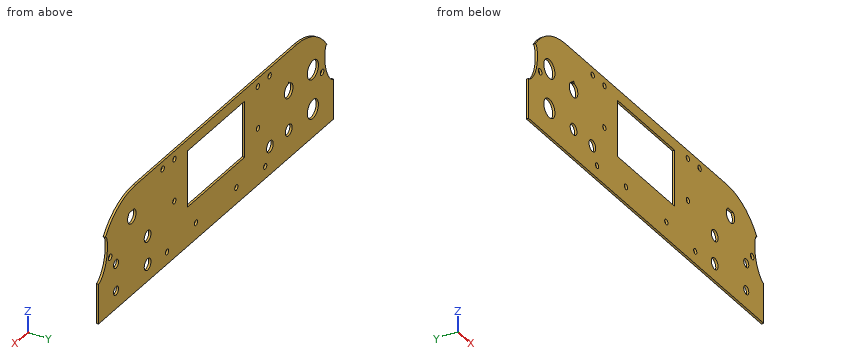
from build123d import *

# Parameters (mm, degrees)
BOSS_EXTRUDE1_DEPTH = 2.54
SKETCH2_W           = 107.95
SKETCH2_H           = 63.5
CUT_EXTRUDE1_DEPTH  = 238.771783963
CUT_EXTRUDE4_START  = -2.54
CUT_EXTRUDE4_DEPTH  = 2.54
SKETCH4_R           = 4.7625
SKETCH4_R_2         = 6.35
SKETCH4_R_3         = 10.5
SKETCH4_R_4         = 3.025
CUT_EXTRUDE3_DEPTH  = 238.771784093
SKETCH6_R           = 3.013751163
SKETCH6_R_2         = 3.176772659
SKETCH6_R_3         = 3.378822927
CUT_EXTRUDE5_DEPTH  = 238.771784093


with BuildPart() as part:
    # Sketch1 → Boss-Extrude1 (new body)
    with BuildSketch(Plane(origin=(0, 0, 0), x_dir=(1, 0, 0), z_dir=(0, 1, 0))):
        with BuildLine():
            Line((222.25, -14.612459999), (222.25, 36.187540001))
            Line((222.25, 36.187540001), (-222.25, 36.187540001))
            Line((-222.25, 36.187540001), (-222.25, -14.612459999))
            ThreePointArc((-222.25, -14.612459999), (-201.791408666, -64.003868664), (-152.4, -84.462459999))
            Line((-152.4, -84.462459999), (152.4, -84.462459999))
            ThreePointArc((152.4, -84.462459999), (201.791408666, -64.003868664), (222.25, -14.612459999))
        make_face()
    extrude(amount=BOSS_EXTRUDE1_DEPTH)

    # Sketch2 → Cut-Extrude1 (cut, through all)
    with BuildSketch(Plane(origin=(0, 2.54, 0), x_dir=(1, 0, 0), z_dir=(0, 1, 0))):
        with Locations((0, -40.012459999)):
            Rectangle(SKETCH2_W, SKETCH2_H)
    extrude(amount=-CUT_EXTRUDE1_DEPTH, mode=Mode.SUBTRACT)

    # Sketch5 → Cut-Extrude4 (cut)
    with BuildSketch(Plane(origin=(0, 2.54, 0), x_dir=(1, 0, 0), z_dir=(0, 1, 0)).offset(CUT_EXTRUDE4_START)):
        with BuildLine():
            ThreePointArc((-222.25, -14.612459999), (-218.970589391, -35.763798683), (-209.440289817, -54.929055063))
            add(Edge.make_bspline(
                [(-209.440289817, -54.929055063), (-204.823931799, -55.506078622), (-202.304901657, -25.266816537), (-219.26819847, -8.373976847), (-222.25, -8.829558466)],
                knots=[0, 0, 0, 0, 0.32580352, 0.516674914, 0.516674914, 0.516674914, 0.516674914], degree=3))
            Line((-222.25, -8.829558466), (-222.25, -14.612459999))
        make_face()
        with BuildLine():
            add(Edge.make_bspline(
                [(-222.25, -8.829558466), (-229.800526338, -9.983183543), (-216.288594077, -54.073048471), (-209.440289817, -54.929055063)],
                knots=[0.516674914, 0.516674914, 0.516674914, 0.516674914, 1, 1, 1, 1], degree=3))
            ThreePointArc((-209.440289817, -54.929055063), (-218.970589391, -35.763798683), (-222.25, -14.612459999))
            Line((-222.25, -14.612459999), (-222.25, -8.829558466))
        make_face()
        with BuildLine():
            add(Edge.make_bspline(
                [(209.440289817, -54.929055063), (204.823931799, -55.506078622), (202.304901657, -25.266816537), (235.136564978, 7.428480335), (216.288594077, -54.073048471), (209.440289817, -54.929055063)],
                knots=[0, 0, 0, 0, 0.32580352, 0.516674914, 1, 1, 1, 1], degree=3))
        make_face()
    extrude(amount=CUT_EXTRUDE4_DEPTH, mode=Mode.SUBTRACT)

    # Sketch4 → Cut-Extrude3 (cut, through all)
    with BuildSketch(Plane(origin=(0, 2.54, 0), x_dir=(1, 0, 0), z_dir=(0, 1, 0))):
        with Locations(Location((189.23, 15.867540001, 0), (0, 0, 270))):
            Circle(SKETCH4_R)
        with Locations(Location((-137.16, 4.437540001, 0), (0, 0, 270))):
            Circle(SKETCH4_R_2)
        with Locations(Location((129.54, 17.137540001, 0), (0, 0, 270))):
            Circle(SKETCH4_R_2)
        with Locations(Location((129.54, -14.612459999, 0), (0, 0, 270))):
            Circle(SKETCH4_R_2)
        with Locations(Location((189.23, -14.612459999, 0), (0, 0, 270))):
            Circle(SKETCH4_R)
        with Locations(Location((-182.88, -40.012459999, 0), (0, 0, 270))):
            Circle(SKETCH4_R_3)
        with Locations(Location((-182.88, 4.437540001, 0), (0, 0, 270))):
            Circle(SKETCH4_R_3)
        with Locations(Location((-101.6, 4.437540001, 0), (0, 0, 270))):
            Circle(SKETCH4_R_2)
        with Locations(Location((-38.130967929, 17.745240001, 0), (0, 0, 270))):
            Circle(SKETCH4_R_4)
        with Locations(Location((-79, -27.947459999, 0), (0, 0, 270))):
            Circle(SKETCH4_R_4)
        with Locations(Location((-78.7827, -75.287459999, 0), (0, 0, 270))):
            Circle(SKETCH4_R_4)
        with Locations(Location((78.7827, -75.287459999, 0), (0, 0, 270))):
            Circle(SKETCH4_R_4)
        with Locations(Location((79, -27.947459999, 0), (0, 0, 270))):
            Circle(SKETCH4_R_4)
        with Locations(Location((38.130967929, 17.745240001, 0), (0, 0, 270))):
            Circle(SKETCH4_R_4)
        with BuildLine():
            Line((-138.01, -48.067737772), (-138.01, -49.812459999))
            Line((-138.01, -49.812459999), (-136.31, -49.812459999))
            Line((-136.31, -49.812459999), (-136.31, -48.067737772))
            ThreePointArc((-136.31, -48.067737772), (-137.16, -31.912459999), (-138.01, -48.067737772))
        make_face()
        with BuildLine():
            Line((164.1475, -59.062459999), (154.6225, -59.062459999))
            ThreePointArc((154.6225, -59.062459999), (159.385, -44.774959999), (164.1475, -59.062459999))
        make_face()
    extrude(amount=-CUT_EXTRUDE3_DEPTH, mode=Mode.SUBTRACT)

    # Sketch6 → Cut-Extrude5 (cut, through all)
    with BuildSketch(Plane.XZ):
        with Locations(Location((92.768348893, -22.335077387, 0), (0, 0, 270))):
            Circle(SKETCH6_R)
        with Locations(Location((101.056164591, 75.862981341, 0), (0, 0, 270))):
            Circle(SKETCH6_R_2)
        with Locations(Location((200.350154748, 27.883658386, 0), (0, 0, 270))):
            Circle(SKETCH6_R_3)
        with Locations(Location((-92.768348893, -22.335077387, 0), (0, 0, 90))):
            Circle(SKETCH6_R)
        with Locations(Location((-200.350154748, 27.883658386, 0), (0, 0, 90))):
            Circle(SKETCH6_R_3)
        with Locations(Location((-101.056164591, 75.862981341, 0), (0, 0, 90))):
            Circle(SKETCH6_R_2)
    extrude(amount=-CUT_EXTRUDE5_DEPTH, mode=Mode.SUBTRACT)


solid = part.part
Source: CAD feature listing. Evaluate the final solid. Frame: model axes, mm. Round coordinates to 2 decimals unless told otherwise and drop trailing zeros. Write each loop counter-clockwise with the first axis right and the second up, starting at its lowest first coordinate (ties: lowest second). Pieces come first, ordered by that corner, then holes. Notation, with made-up numbers: (50.25, 45) - (79.25, 45) arc R20 cw to (79.25, 49) - close; hole circle Ø8 at (1, 74.25). An arc over 180 degrees is marked (long way). Use CSV: the item, a comma, the result in double quotes. Start each with the question number.
(1) Cut plane A-A, the plane x = 189.23. Return loops of the section in (y, z), and give its area (3 significant figures).
(2) Material intervals for probe 1 along Z at (x, y) = (-142, 0.1); probe 2 along X at (y, z) = (2.25, 15) (3 decimals); probe 3 along Z at (x, y) = (-43, 0.95), sorted ascending. Write a range as [from, to].
(3) Cut plane C-C, the plane y = 0.9. Give the number of separate pieces and of enclosed holes in the cut face, and give its area (3 significant figures).
(4) Cut plane B-B, the plane x = -182.88. Return loops of the section in (y, z).
(5) First-contact query: pin 1 Ø0.9 at (y, z) = (2, 49) entering from +X. Flat tip, straight axial feed; report the tip coordinate or a pass-through.
Geometry says:
1,outline,"(0, -36.19) - (2.54, -36.19) - (2.54, -20.63) - (0, -20.63) - close; (0, -11.11) - (2.54, -11.11) - (2.54, 9.85) - (0, 9.85) - close; (0, 19.37) - (2.54, 19.37) - (2.54, 73.96) - (0, 73.96) - close"
1,area,"231 mm²"
2,probe 1,"[-36.19, -8.55], [-0.33, 33.52], [46.51, 84.46]"
2,probe 2,"[-213.973, -53.975], [53.975, 123.202], [135.878, 184.483], [193.977, 213.973]"
2,probe 3,"[-36.19, 8.26], [71.76, 84.46]"
3,separate pieces,"1"
3,enclosed holes,"23"
3,area,"41,700 mm²"
4,outline,"(0, -36.19) - (2.54, -36.19) - (2.54, -14.94) - (0, -14.94) - close; (0, 6.06) - (2.54, 6.06) - (2.54, 29.51) - (0, 29.51) - close; (0, 50.51) - (2.54, 50.51) - (2.54, 77.46) - (0, 77.46) - close"
5,pin 1,"x = 205.92"
